from build123d import *

# Parameters (mm, degrees)
BOSS_EXTRU_1_DEPTH      = 3
D_GAGEMENT_M41_D        = 4.5
D_GAGEMENT_M41_DEPTH    = 10
D_GAGEMENT_M41_TIP      = 1.351936393
D_GAGEMENT_M201_D       = 22
D_GAGEMENT_M201_DEPTH   = 10
D_GAGEMENT_M201_TIP     = 6.609466809
D_GAGEMENT_M32_D        = 3.4
D_GAGEMENT_M32_DEPTH    = 10
D_GAGEMENT_M32_TIP      = 1.021463052
D_GAGEMENT_M43_D        = 4.5
ESQUISSE27_W            = 35
ESQUISSE27_H            = 15
ENL_V_MAT_EXTRU_2_DEPTH = 4
D_GAGEMENT_M33_D        = 3.4
D_GAGEMENT_M33_DEPTH    = 7.01
D_GAGEMENT_M33_TIP      = 1.021463052


with BuildPart() as part:
    # Esquisse1 → Boss.-Extru.1 (new body)
    with BuildSketch(Plane.XY):
        with BuildLine():
            Line((-145, 85), (-109.886246, 120.113754))
            Line((-109.886246, 120.113754), (-104.886246, 120.113754))
            ThreePointArc((-104.886246, 120.113754), (0, 20), (104.886246, 120.113754))
            Line((104.886246, 120.113754), (109.886246, 120.113754))
            Line((109.886246, 120.113754), (145, 85))
            Line((145, 85), (145, 37.5))
            Line((145, 37.5), (120, 37.5))
            Line((120, 37.5), (120, -37.5))
            Line((120, -37.5), (145, -37.5))
            Line((145, -37.5), (145, -85))
            Line((145, -85), (109.886246, -120.113754))
            Line((109.886246, -120.113754), (104.886246, -120.113754))
            ThreePointArc((104.886246, -120.113754), (0, -20), (-104.886246, -120.113754))
            Line((-104.886246, -120.113754), (-109.886246, -120.113754))
            Line((-109.886246, -120.113754), (-145, -85))
            Line((-145, -85), (-145, -37.5))
            Line((-145, -37.5), (-120, -37.5))
            Line((-120, -37.5), (-120, 37.5))
            Line((-120, 37.5), (-145, 37.5))
            Line((-145, 37.5), (-145, 85))
        make_face()
    extrude(amount=BOSS_EXTRU_1_DEPTH)

    # Dégagement M41
    with Locations(Plane(origin=(-139.3, 79.3, 3), x_dir=(1, 0, 0), z_dir=(0, 0, 1))):
        with Locations((0, 0), (278.6, 0), (278.6, -158.6), (0, -158.6)):
            Hole(D_GAGEMENT_M41_D / 2, depth=D_GAGEMENT_M41_DEPTH)
            with Locations((0, 0, -(D_GAGEMENT_M41_DEPTH + D_GAGEMENT_M41_TIP / 2))):  # 118° drill point
                Cone(0, D_GAGEMENT_M41_D / 2, D_GAGEMENT_M41_TIP, mode=Mode.SUBTRACT)

    # Dégagement M201
    with Locations(Plane(origin=(-115, 80.113754, 3), x_dir=(1, 0, 0), z_dir=(0, 0, 1))):
        with Locations((0, 0), (230, 0), (230, -160.227508), (0, -160.227508)):
            Hole(D_GAGEMENT_M201_D / 2, depth=D_GAGEMENT_M201_DEPTH)
            with Locations((0, 0, -(D_GAGEMENT_M201_DEPTH + D_GAGEMENT_M201_TIP / 2))):  # 118° drill point
                Cone(0, D_GAGEMENT_M201_D / 2, D_GAGEMENT_M201_TIP, mode=Mode.SUBTRACT)

    # Dégagement M32
    with Locations(Plane.XY.offset(3)):
        with Locations((-103.741669751, 73.613754), (-115, 93.113754), (-126.258330249, 73.613754), (-103.741669751, -73.613754), (-126.258330249, -73.613754), (-115, -93.113754), (115, -93.113754), (126.258330249, -73.613754), (103.741669751, -73.613754), (103.741669751, 73.613754), (115, 93.113754), (126.258330249, 73.613754)):
            Hole(D_GAGEMENT_M32_D / 2, depth=D_GAGEMENT_M32_DEPTH)
            with Locations((0, 0, -(D_GAGEMENT_M32_DEPTH + D_GAGEMENT_M32_TIP / 2))):  # 118° drill point
                Cone(0, D_GAGEMENT_M32_D / 2, D_GAGEMENT_M32_TIP, mode=Mode.SUBTRACT)

    # Dégagement M43 (through all)
    with Locations(Plane.XY.offset(3)):
        with Locations((-110, -32.5), (-90, -32.5), (-67.5, -13), (-67.5, 7.5), (-67.5, 28), (67.5, 28), (67.5, 7.5), (67.5, -13), (90, -32.5), (110, -32.5)):
            Hole(D_GAGEMENT_M43_D / 2)

    # Esquisse27 → Enlèv. mat.-Extru.2 (cut, through all)
    with BuildSketch(Plane(origin=(0, 0, 0), x_dir=(-1, 0, 0), z_dir=(0, 0, -1))):
        with Locations((-115, 52.5)):
            Rectangle(ESQUISSE27_W, ESQUISSE27_H)
        with Locations((-115, -52.5)):
            Rectangle(ESQUISSE27_W, ESQUISSE27_H)
        with Locations((115, -52.5)):
            Rectangle(ESQUISSE27_W, ESQUISSE27_H)
        with Locations((115, 52.5)):
            Rectangle(ESQUISSE27_W, ESQUISSE27_H)
    extrude(amount=-ENL_V_MAT_EXTRU_2_DEPTH, mode=Mode.SUBTRACT)

    # Dégagement M33
    with Locations(Plane(origin=(0, 0, 0), x_dir=(-1, 0, 0), z_dir=(0, 0, -1))):
        with Locations((-137.5, 52.5), (-92.5, 52.5), (-137.5, -52.5), (-92.5, -52.5), (92.5, 52.5), (137.5, 52.5), (92.5, -52.5), (137.5, -52.5)):
            Hole(D_GAGEMENT_M33_D / 2, depth=D_GAGEMENT_M33_DEPTH)
            with Locations((0, 0, -(D_GAGEMENT_M33_DEPTH + D_GAGEMENT_M33_TIP / 2))):  # 118° drill point
                Cone(0, D_GAGEMENT_M33_D / 2, D_GAGEMENT_M33_TIP, mode=Mode.SUBTRACT)


solid = part.part
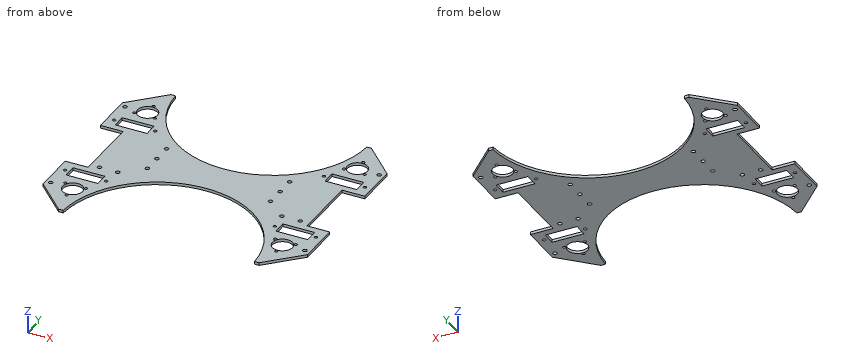
Work out the finished part from the listing and answer in its coordinate system (mm). Coordinates: 2 decimals unless noted, no trailing zeros. Loops run counter-clockwise (first coordinate to the right, second up) from the corner with the lowest first, then second, coordinate; pieces in that order, holes last. Notation, with made-up numbers: (-38, 44) -> (4, 44) arc R22 ccw to (4, 52) -> close; hole circle Ø4 at (-7, -8.75). An arc over 180 degrees is marked (long way). Write each question's results on one line, items separated by ' | '. Start each with the question number.
1) Flat-ended cylindrical pins translate along their axes: P1, Ø5.5, axis at x = -115, y = -93.11, coming from the +Z side; P2, Ø1, axis at y = -23, z = 1, coming from the -X side. Find the tip coordinate at first contact, or state that the pin passes through.
2) Find section A-A on y = -24. Determine the outline of the cut face in (x, z).
3) Consider line 1 along Y through (x, z) = (92.5, 1.3); line 2 along X through (y, z) = (-48.5, 1.5); line 3 along Y through (x, z) = (93, 0.85). Determine where each line is inside the solid, lowest interval first.
4) Find section B-B on y = 65. Determine the outline of the cut face in (x, z).
5) Find section C-C on x = -73. Determine the outline of the cut face in (y, z), then the cut area to 3 significant figures.
6) Find section D-D on z = 0.6. Count the separate pieces of the cut face and the enclosed holes in it, then the cut area to 3 significant figures.
Response values:
1) P1: stops at z = 3 | P2: stops at x = -120
2) outline: (-120, 0) -> (-28.71, 0) -> (-28.71, 3) -> (-120, 3) -> close; (28.71, 0) -> (120, 0) -> (120, 3) -> (28.71, 3) -> close
3) line 1: y = -75.31 to -54.2, -50.8 to 50.8, 54.2 to 75.31 | line 2: x = -145 to -132.5, -97.5 to -71.92, 71.92 to 97.5, 132.5 to 145 | line 3: y = -76.26 to -54.12, -50.88 to 50.88, 54.12 to 76.26
4) outline: (-145, 0) -> (-86.17, 0) -> (-86.17, 3) -> (-145, 3) -> close; (86.17, 0) -> (145, 0) -> (145, 3) -> (86.17, 3) -> close
5) outline: (-49.53, 0) -> (49.53, 0) -> (49.53, 3) -> (-49.53, 3) -> close | area: 297 mm^2
6) separate pieces: 1 | enclosed holes: 42 | area: 26,800 mm^2
